```python
from build123d import *

# Parameters (mm, degrees)
SCHIZZO1_W                   = 33
SCHIZZO1_H                   = 22.5
SCHIZZO1_W_2                 = 23
SCHIZZO1_H_2                 = 12.5
ESTRUSIONE_ESTRUSIONE1_DEPTH = 2.35
SCHIZZO2_R                   = 1
TAGLIO_ESTRUSIONE1_DEPTH     = 2.35
SPECCHIA2_COPY_1_SKETCH_R    = 1
SPECCHIA2_COPY_1_DEPTH       = 2.35
SCHIZZO3_R                   = 1
TAGLIO_ESTRUSIONE2_DEPTH     = 2.35


with BuildPart() as part:
    # Schizzo1 → Estrusione-Estrusione1 (new body)
    with BuildSketch(Plane.XY):
        Rectangle(SCHIZZO1_W, SCHIZZO1_H)
        Rectangle(SCHIZZO1_W_2, SCHIZZO1_H_2, mode=Mode.SUBTRACT)
    extrude(amount=ESTRUSIONE_ESTRUSIONE1_DEPTH)

    # Schizzo2 → Taglio-Estrusione1 (cut)
    with BuildSketch(Plane.XY.offset(2.35)):
        with Locations((-14, 8.5)):
            Circle(SCHIZZO2_R)
    taglio_estrusione1 = extrude(amount=-TAGLIO_ESTRUSIONE1_DEPTH, mode=Mode.SUBTRACT)

    # Specchia1: Taglio-Estrusione1 across plane
    add(taglio_estrusione1.mirror(Plane.ZX), mode=Mode.SUBTRACT)

    # Specchia2: Taglio-Estrusione1 across plane
    add(taglio_estrusione1.mirror(Plane(origin=(0, 0, 0), x_dir=(0, 0, 1), z_dir=(1, 0, 0))), mode=Mode.SUBTRACT)

    # Specchia2 copy 1 sketch → Specchia2 copy 1 (cut)
    with BuildSketch(Plane(origin=(0, 0, 2.35), x_dir=(-1, 0, 0), z_dir=(0, 0, 1))):
        with Locations((-14, 8.5)):
            Circle(SPECCHIA2_COPY_1_SKETCH_R)
    extrude(amount=-SPECCHIA2_COPY_1_DEPTH, mode=Mode.SUBTRACT)

    # Schizzo3 → Taglio-Estrusione2 (cut)
    with BuildSketch(Plane.XY.offset(2.35)):
        with Locations((14.475, 0)):
            Circle(SCHIZZO3_R)
    taglio_estrusione2 = extrude(amount=-TAGLIO_ESTRUSIONE2_DEPTH, mode=Mode.SUBTRACT)

    # Specchia3: Taglio-Estrusione2 across plane
    add(taglio_estrusione2.mirror(Plane(origin=(0, 0, 0), x_dir=(0, 0, 1), z_dir=(1, 0, 0))), mode=Mode.SUBTRACT)


solid = part.part
```
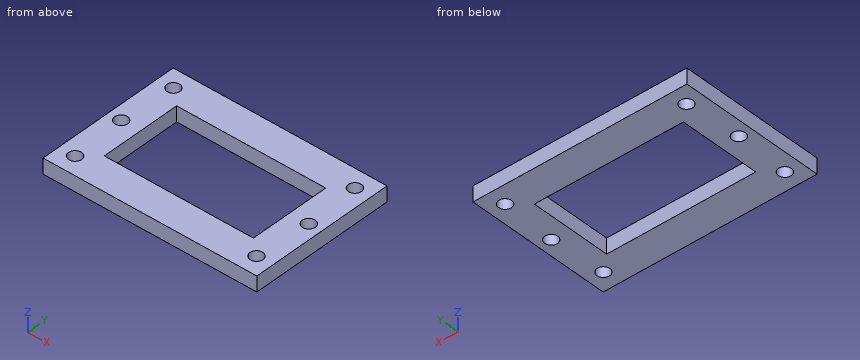
Can you work these out from the model? Positions are in its coordinate system, mm. Round coordinates to 2 decimals unless told otherwise and drop trailing zeros. Loops run counter-clockwise (first coordinate to the right, second up) from the corner with the lowest first, then second, coordinate; pieces in that order, holes last. Notation, with made-up numbers: (63, 65) -> (118, 65) arc R22 ccw to (118, 99) -> close; hole circle Ø10 at (13.5, -9). An arc over 180 degrees is marked (long way). One line per item, written item: value. Start each with the question number.
1. If we section it at D-D, the plane x = -14: Write out the boundary of the cut face in (y, z), then the cut area to 3 significant figures.
2. If I drill on probe 1 along X at (y, z) = (-8.5, 0.95); probe 2 along Y at (x, z) = (-11, 1.1); probe 3 along Y at (x, z) = (14, 0.95), over which ranges is the centre line in solid material (lowest first)?
3. If we section it at A-A, the plane y = -5.25: Write out the boundary of the cut face in (x, z), then the cut area to 3 significant figures.
4. For pin 1 (1.8 mm diameter, centred on x = -14, y = 8.5, fed in from +Z), with a flat end and sliding along its axis, tell me the tip position at first contact or that it passes through.
5. If we section it at B-B, the plane x = 1.5: Write out the boundary of the cut face in (y, z).
6. If we section it at C-C, the plane z = 1.1: Write out the boundary of the cut face in (x, y) (3 decimals).
Calculated:
1. outline: (-11.25, 0) -> (-9.5, 0) -> (-9.5, 2.35) -> (-11.25, 2.35) -> close; (-7.5, 0) -> (-0.88, 0) -> (-0.88, 2.35) -> (-7.5, 2.35) -> close; (0.88, 0) -> (7.5, 0) -> (7.5, 2.35) -> (0.88, 2.35) -> close; (9.5, 0) -> (11.25, 0) -> (11.25, 2.35) -> (9.5, 2.35) -> close
1. area: 39.3 mm²
2. probe 1: x = -16.5 to -15, -13 to 13, 15 to 16.5
2. probe 2: y = -11.25 to -6.25, 6.25 to 11.25
2. probe 3: y = -11.25 to -9.5, -7.5 to -0.88, 0.88 to 7.5, 9.5 to 11.25
3. outline: (-16.5, 0) -> (-11.5, 0) -> (-11.5, 2.35) -> (-16.5, 2.35) -> close; (11.5, 0) -> (16.5, 0) -> (16.5, 2.35) -> (11.5, 2.35) -> close
3. area: 23.5 mm²
4. pin 1: passes through
5. outline: (-11.25, 0) -> (-6.25, 0) -> (-6.25, 2.35) -> (-11.25, 2.35) -> close; (6.25, 0) -> (11.25, 0) -> (11.25, 2.35) -> (6.25, 2.35) -> close
6. outline: (-16.5, -11.25) -> (16.5, -11.25) -> (16.5, 11.25) -> (-16.5, 11.25) -> close; hole circle Ø2 at (-14.475, 0); hole circle Ø2 at (-14, -8.5); hole circle Ø2 at (-14, 8.5); hole (-11.5, -6.25) -> (11.5, -6.25) -> (11.5, 6.25) -> (-11.5, 6.25) -> close; hole circle Ø2 at (14, -8.5); hole circle Ø2 at (14, 8.5); hole circle Ø2 at (14.475, 0)
